Read the model definition and answer for the solid it produces. Units are mm, in the model's axes. Give positions to 0.01 mm unless a question says otherwise; leave off trailing zeros. Order: outer loops, then holes, each group sorted by start corner. A loop starts at its lowest first (then second) coordinate and runs counter-clockwise, first axis right, second up. Notation, with made-up numbers: (6, 8) -> (59, 8) arc R34 cw to (59, 47) -> close; hole circle Ø6 at (27.25, 36). An arc over 180 degrees is marked (long way). Answer as CSV lines item,"result". Start each with the question number.
1) Find section B-B (y = 29.5). Determine the outline of the cut face in (x, z).
2) A flat-ended cylindrical pin translates along its axis: pin 1 Ø2 at (y, z) = (24.5, 3) entering from +X. Find the tip coordinate at first contact, or state that the pin passes through.
3) The mould has two halves that part along X. Classify faces 1 (the face through (-9, 38.414, 2)), 2 (the face through (-59.758, -1, 2)), 3 (the face through (50.37, 13.27, 2.46)): +X half, -X half, draft (parallel to the pull), parting line (faces both ways), or undercut.
4) Straight lines are drawn through the part: L1, parallel to X at y = 5, z = 0.9; L2, parallel to X at y = 13, z = 1.35; L3, parallel to Y at x = -55, z = 0.5. For each, find the intervals that lie inside material, in ascending order. Write a range as from..to.
```python
from build123d import *

# Parameters (mm, degrees)
F1_DEPTH = 5


with BuildPart() as f1:
    # F0 (on Top) → F1 (new body)
    with BuildSketch(Plane.XY):
        with BuildLine():
            Line((-9.758077, 38.413576), (-59.758077, 38.413576))
            Line((-59.758077, 38.413576), (-59.758077, 19.413576))
            Line((-59.758077, 19.413576), (-59.758077, 17.216746))
            ThreePointArc((-59.758077, 17.216746), (-59.229749, 15.942835), (-57.954909, 15.416749))
            Line((-57.954909, 15.416749), (-57.085515, 15.41643))
            ThreePointArc((-57.085515, 15.41643), (-49.623063, 13.411928), (-57.087164, 11.413576))
            Line((-57.087164, 11.413576), (-57.948048, 11.413576))
            Line((-57.948048, 11.413576), (-57.954909, 11.410403))
            ThreePointArc((-57.954909, 11.410403), (-59.229749, 10.884318), (-59.758077, 9.610406))
            Line((-59.758077, 9.610406), (-59.758077, 7.413576))
            Line((-59.758077, 7.413576), (-59.758077, -11.586424))
            Line((-59.758077, -11.586424), (-9.758077, -11.586424))
            Line((-9.758077, -11.586424), (-9.758077, 7.413576))
            Line((-9.758077, 7.413576), (-9.758077, 9.610406))
            ThreePointArc((-9.758077, 9.610406), (-9.229749, 10.884318), (-7.954909, 11.410403))
            Line((-7.954909, 11.410403), (-7.948048, 11.413576))
            Line((-7.948048, 11.413576), (-7.087164, 11.413576))
            ThreePointArc((-7.087164, 11.413576), (0.376937, 13.411928), (-7.085515, 15.41643))
            Line((-7.085515, 15.41643), (-7.954909, 15.416749))
            ThreePointArc((-7.954909, 15.416749), (-9.229749, 15.942835), (-9.758077, 17.216746))
            Line((-9.758077, 17.216746), (-9.758077, 19.413576))
            Line((-9.758077, 19.413576), (-9.758077, 38.413576))
        make_face()
        with BuildLine():
            Line((40.241923, 38.413576), (-9.758077, 38.413576))
            Line((-9.758077, 38.413576), (-9.758077, 19.413576))
            Line((-9.758077, 19.413576), (-9.758077, 17.216746))
            ThreePointArc((-9.758077, 17.216746), (-9.229749, 15.942835), (-7.954909, 15.416749))
            Line((-7.954909, 15.416749), (-7.085515, 15.41643))
            ThreePointArc((-7.085515, 15.41643), (0.376937, 13.411928), (-7.087164, 11.413576))
            Line((-7.087164, 11.413576), (-7.948048, 11.413576))
            Line((-7.948048, 11.413576), (-7.954909, 11.410403))
            ThreePointArc((-7.954909, 11.410403), (-9.229749, 10.884318), (-9.758077, 9.610406))
            Line((-9.758077, 9.610406), (-9.758077, 7.413576))
            Line((-9.758077, 7.413576), (-9.758077, -11.586424))
            Line((-9.758077, -11.586424), (40.241923, -11.586424))
            Line((40.241923, -11.586424), (40.241923, 9.613576))
            ThreePointArc((40.241923, 9.613576), (40.769131, 10.886368), (42.041923, 11.413576))
            Line((42.041923, 11.413576), (42.907822, 11.413576))
            ThreePointArc((42.907822, 11.413576), (50.371923, 13.413576), (42.907822, 15.413576))
            Line((42.907822, 15.413576), (42.041923, 15.413576))
            ThreePointArc((42.041923, 15.413576), (40.769131, 15.940784), (40.241923, 17.213576))
            Line((40.241923, 17.213576), (40.241923, 38.413576))
        make_face()
    extrude(amount=F1_DEPTH)


solid = f1.part
```
Findings below:
1,outline,"(-59.76, 0) -> (40.24, 0) -> (40.24, 5) -> (-59.76, 5) -> close"
2,pin 1,"x = 40.24"
3,face 1,"draft"
3,face 2,"-X half"
3,face 3,"undercut"
4,L1,"-59.76..40.24"
4,L2,"-49.64..50.35"
4,L3,"-11.59..9.66, 17.17..38.41"
